Can you work these out from the model? Positions are in its coordinate system, mm. Face numbers are marked on the shaded views. A direction names the side the tool comes from. Give positions to 0.01 mm unless a question says otherwise; leave off trailing zeros. Order: outer loops, then holes, each group sorted by start corner. A loop starts at its lowest first (then second) coordinate and runs counter-clockwise, first axis right, second up. Notation, with made-up numbers: (39, 57.5) - (47, 57.5) arc R12 ccw to (47, 70.5) - close; hole circle Ø5 at (26.5, 30.5). An arc over 180 degrees is marked (long way). Write each question's results on one line, items separated by ' | '. Start each with the question number.
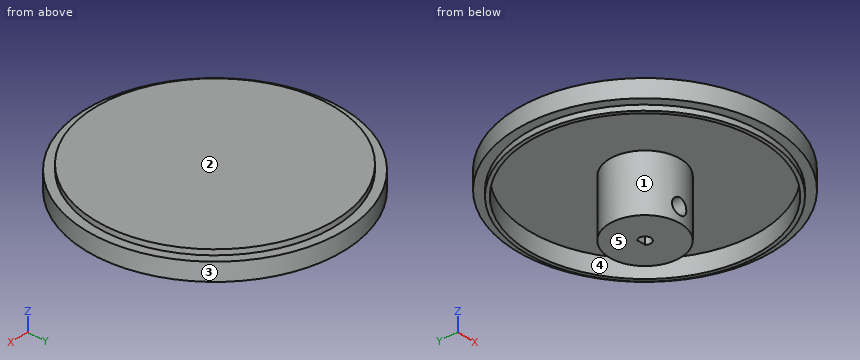
from build123d import *

# Parameters (mm, degrees)
ESBO_O1_R                     = 35
ESBO_O1_R_2                   = 32.5
RESSALTO_EXTRUS_O1_DEPTH      = 8
RESSALTO_EXTRUS_O2_START      = -3
ESBO_O2_R                     = 32.5
RESSALTO_EXTRUS_O2_DEPTH      = 3
ESBO_O3_R                     = 2.5
CORTE_EXTRUS_O1_DEPTH         = 3
RESSALTO_EXTRUS_O3_DEPTH      = 5
RESSALTO_EXTRUS_O3_DEPTH_BACK = 3
ESBO_O4_R                     = 37
ESBO_O4_R_2                   = 35
ESBO_O5_W                     = 1.8
ESBO_O5_H                     = 3
ESBO_O6_R                     = 12.55
RESSALTO_EXTRUS_O4_DEPTH      = 5
CORTE_EXTRUS_O2_DEPTH         = 53.933921071
CORTE_EXTRUS_O2_DEPTH_BACK    = 53.933921071
ESBO_O7_R                     = 7.55
RESSALTO_EXTRUS_O5_START      = -8
ESBO_O8_R                     = 37
ESBO_O8_R_2                   = 32.5
RESSALTO_EXTRUS_O5_DEPTH      = 8
ESBO_O9_R                     = 37
ESBO_O9_R_2                   = 33.5
CORTE_EXTRUS_O8_DEPTH         = 1.5
CORTE_EXTRUS_O9_START         = -1.5
ESBO_O12_R                    = 37
ESBO_O12_R_2                  = 33.5
CORTE_EXTRUS_O9_DEPTH         = 1.5
CORTE_EXTRUS_O10_START        = -10
ESBO_O13_R                    = 37
ESBO_O13_R_2                  = 36
CORTE_EXTRUS_O10_DEPTH        = 10
ESBO_O14_R                    = 37
ESBO_O14_R_2                  = 36
RESSALTO_EXTRUS_O6_DEPTH      = 5
ESBO_O15_R                    = 12.55
CORTE_EXTRUS_O11_DEPTH        = 53.933921071
ESBO_O16_R                    = 12.55
RESSALTO_EXTRUS_O7_DEPTH      = 3
ESBO_O17_R                    = 10
RESSALTO_EXTRUS_O8_DEPTH      = 16
ESBO_O18_R                    = 3.3
CORTE_EXTRUS_O12_DEPTH        = 16
ESBO_O23_R                    = 37
ESBO_O23_R_2                  = 36
CORTE_EXTRUS_O15_DEPTH        = 54.798234172
ESBO_O24_R                    = 3.3
RESSALTO_EXTRUS_O9_DEPTH      = 11
CORTE_EXTRUS_O14_DEPTH        = 56.88103435
CORTE_EXTRUS_O14_DEPTH_BACK   = 56.88103435
ESBO_O21_R                    = 2.2


with BuildPart() as part:
    # Esboço1 → Ressalto-extrusão1 (new body)
    with BuildSketch(Plane.XY):
        Circle(ESBO_O1_R)
        Circle(ESBO_O1_R_2, mode=Mode.SUBTRACT)
    extrude(amount=RESSALTO_EXTRUS_O1_DEPTH)

    # Esboço2 → Ressalto-extrusão2 (add)
    with BuildSketch(Plane.XY.offset(8).offset(RESSALTO_EXTRUS_O2_START)):
        Circle(ESBO_O2_R)
    extrude(amount=RESSALTO_EXTRUS_O2_DEPTH)

    # Esboço3 → Corte-extrusão1 (cut)
    with BuildSketch(Plane.XY.offset(8)):
        Circle(ESBO_O3_R)
    extrude(amount=-CORTE_EXTRUS_O1_DEPTH, mode=Mode.SUBTRACT)

    # Esboço4 → Ressalto-extrusão3 (add, two sides: drawn at the far end of the back side and taken through both)
    with BuildSketch(Plane(origin=(0, 0, 5), x_dir=(-1, 0, 0), z_dir=(0, 0, -1)).offset(-RESSALTO_EXTRUS_O3_DEPTH_BACK)):
        Circle(ESBO_O4_R)
        Circle(ESBO_O4_R_2, mode=Mode.SUBTRACT)
    extrude(amount=RESSALTO_EXTRUS_O3_DEPTH + RESSALTO_EXTRUS_O3_DEPTH_BACK)

    # Esboço5 → Corte-Revolução1 (revolve, cut)
    with BuildSketch(Plane(origin=(0, 0, 0), x_dir=(1, 0, 0), z_dir=(0, 1, 0))):
        with Locations((-36.1, -2.5)):
            Rectangle(ESBO_O5_W, ESBO_O5_H)
        with Locations((-36.1, -5.5)):
            Rectangle(ESBO_O5_W, ESBO_O5_H)
    revolve(axis=Axis((0, 0, 8), (0, 0, -1)), mode=Mode.SUBTRACT)

    # Esboço6 → Ressalto-extrusão4 (add)
    with BuildSketch(Plane(origin=(0, 0, 5), x_dir=(-1, 0, 0), z_dir=(0, 0, -1))):
        with Locations(Location((0, 0, 0), (0, 0, 180))):
            Circle(ESBO_O6_R)
    extrude(amount=RESSALTO_EXTRUS_O4_DEPTH)

    # Esboço7 → Corte-extrusão2 (cut, two sides: drawn at the far end of the back side and taken through both)
    with BuildSketch(Plane(origin=(0, 0, 0), x_dir=(-1, 0, 0), z_dir=(0, 0, -1)).offset(-CORTE_EXTRUS_O2_DEPTH_BACK)):
        Circle(ESBO_O7_R)
    extrude(amount=CORTE_EXTRUS_O2_DEPTH + CORTE_EXTRUS_O2_DEPTH_BACK, mode=Mode.SUBTRACT)

    # Esboço8 → Ressalto-extrusão5 (add)
    with BuildSketch(Plane.XY.offset(8).offset(RESSALTO_EXTRUS_O5_START)):
        with Locations(Location((0, 0, 0), (0, 0, 180))):
            Circle(ESBO_O8_R)
        Circle(ESBO_O8_R_2, mode=Mode.SUBTRACT)
    extrude(amount=RESSALTO_EXTRUS_O5_DEPTH)

    # Esboço9 → Corte-extrusão8 (cut)
    with BuildSketch(Plane.XY.offset(8)):
        with Locations(Location((0, 0, 0), (0, 0, 180))):
            Circle(ESBO_O9_R)
        Circle(ESBO_O9_R_2, mode=Mode.SUBTRACT)
    extrude(amount=-CORTE_EXTRUS_O8_DEPTH, mode=Mode.SUBTRACT)

    # Esboço12 → Corte-extrusão9 (cut)
    with BuildSketch(Plane(origin=(0, 0, 0), x_dir=(-1, 0, 0), z_dir=(0, 0, -1)).offset(CORTE_EXTRUS_O9_START)):
        Circle(ESBO_O12_R)
        with Locations(Location((0, 0, 0), (0, 0, 180))):
            Circle(ESBO_O12_R_2, mode=Mode.SUBTRACT)
    extrude(amount=CORTE_EXTRUS_O9_DEPTH, mode=Mode.SUBTRACT)

    # Esboço13 → Corte-extrusão10 (cut)
    with BuildSketch(Plane(origin=(0, 0, 1.5), x_dir=(-1, 0, 0), z_dir=(0, 0, -1)).offset(CORTE_EXTRUS_O10_START)):
        Circle(ESBO_O13_R)
        Circle(ESBO_O13_R_2, mode=Mode.SUBTRACT)
    extrude(amount=CORTE_EXTRUS_O10_DEPTH, mode=Mode.SUBTRACT)

    # Esboço14 → Ressalto-extrusão6 (add)
    with BuildSketch(Plane.XY.offset(6.5)):
        Circle(ESBO_O14_R)
        Circle(ESBO_O14_R_2, mode=Mode.SUBTRACT)
    extrude(amount=-RESSALTO_EXTRUS_O6_DEPTH)

    # Esboço15 → Corte-extrusão11 (cut, through all)
    with BuildSketch(Plane(origin=(0, 0, 0), x_dir=(-1, 0, 0), z_dir=(0, 0, -1))):
        Circle(ESBO_O15_R)
    extrude(amount=-CORTE_EXTRUS_O11_DEPTH, mode=Mode.SUBTRACT)

    # Esboço16 → Ressalto-extrusão7 (add, through all)
    with BuildSketch(Plane(origin=(0, 0, 5), x_dir=(-1, 0, 0), z_dir=(0, 0, -1))):
        Circle(ESBO_O16_R)
    extrude(amount=-RESSALTO_EXTRUS_O7_DEPTH)

    # Esboço17 → Ressalto-extrusão8 (add)
    with BuildSketch(Plane(origin=(0, 0, 5), x_dir=(-1, 0, 0), z_dir=(0, 0, -1))):
        with Locations(Location((0, 0, 0), (0, 0, 180))):
            Circle(ESBO_O17_R)
    extrude(amount=RESSALTO_EXTRUS_O8_DEPTH)

    # Esboço18 → Corte-extrusão12 (cut)
    with BuildSketch(Plane(origin=(0, 0, -11), x_dir=(-1, 0, 0), z_dir=(0, 0, -1))):
        Circle(ESBO_O18_R)
    extrude(amount=-CORTE_EXTRUS_O12_DEPTH, mode=Mode.SUBTRACT)

    # Esboço23 → Corte-extrusão15 (cut, through all)
    with BuildSketch(Plane(origin=(0, 0, 1.5), x_dir=(-1, 0, 0), z_dir=(0, 0, -1))):
        Circle(ESBO_O23_R)
        Circle(ESBO_O23_R_2, mode=Mode.SUBTRACT)
    extrude(amount=-CORTE_EXTRUS_O15_DEPTH, mode=Mode.SUBTRACT)

    # Esboço24 → Ressalto-extrusão9 (add)
    with BuildSketch(Plane(origin=(0, 0, -11), x_dir=(-1, 0, 0), z_dir=(0, 0, -1))):
        Circle(ESBO_O24_R)
        with BuildLine():
            Line((-1.229837388, 1.1), (1.229837388, 1.1))
            ThreePointArc((1.229837388, 1.1), (0, -1.65), (-1.229837388, 1.1))
        make_face(mode=Mode.SUBTRACT)
    extrude(amount=-RESSALTO_EXTRUS_O9_DEPTH)

    # Esboço21 → Corte-extrusão14 (cut, two sides: drawn at the far end of the back side and taken through both)
    with BuildSketch(Plane(origin=(0, 5.3, 0), x_dir=(1, 0, 0), z_dir=(0, 1, 0)).offset(-CORTE_EXTRUS_O14_DEPTH_BACK)):
        with Locations(Location((0, 6.85, 0), (0, 0, 180))):
            Circle(ESBO_O21_R)
    extrude(amount=CORTE_EXTRUS_O14_DEPTH + CORTE_EXTRUS_O14_DEPTH_BACK, mode=Mode.SUBTRACT)


solid = part.part
Q1. If I drill on probe 1 along Z at (x, y) = (0, 1.75); probe 2 along Y at (x, z) = (0, -1.7); probe 3 along Y at (x, z) = (-5.5, 3.25), over which ranges is the centre line in solid material (lowest first)? Write a range as from..to.
Q2. Thinking about a two-plate mould opening in Y: for the marked faces 1, 2 and 3, which applies, released by +Y, released by -Y, zero draft, split by the parting line, or undercut?
Q3. If we section it at B-B (x = 0): State how many separate pieces and enclosed holes the cut face has, plus the area to 3 significant figures.
Q4. Will these pins go through, and if not, where does the flat tip stop? P1, Ø3, axis at y = -22, z = 4, coming from the -X side; P2, Ø8, axis at x = -17.5, z = 2.5, coming from the -Y side; P3, Ø2.5, axis at x = 0.5, z = -10.5, coming from the -Y side.
Q5. Which directions (+Z, -Z, +X, -X, +Y, -Y) give clear straight access to the entire face, cutting with the end or side of a thin tool? Please do the marked faces 4 and 5.
Q6. If we section it at D-D (x = -12.5): Please give me the cut outline in (y, z).
Q7. If we section it at C-C (z = -1.75): Please give me the cut outline in (x, y), plus the area to 3 significant figures.
Findings below:
1) probe 1: z = -11..-9.05, -4.65..0, 5..8 | probe 2: y = -10..-1.65, 1.1..10 | probe 3: y = -35.58..-32.03, -8.35..8.35, 32.03..35.58
2) face 1: undercut | face 2: zero draft | face 3: split by the parting line
3) separate pieces: 3 | enclosed holes: 0 | area: 417 mm2
4) P1: stops at x = -29.59 | P2: stops at y = -33.37 | P3: stops at y = -10
5) face 4: -Z | face 5: -Z, +X, -X, +Y, -Y
6) outline: (-33.76, 1.5) - (-31.08, 1.5) - (-31.08, 0) - (-30, 0) - (-30, 5) - (30, 5) - (30, 0) - (31.08, 0) - (31.08, 1.5) - (33.76, 1.5) - (33.76, 6.5) - (31.08, 6.5) - (31.08, 8) - (-31.08, 8) - (-31.08, 6.5) - (-33.76, 6.5) - close
7) outline: circle Ø20 at (0, 0); hole (-1.23, 1.1) arc R1.65 ccw (long way) to (1.23, 1.1) - close | area: 307 mm2
